from build123d import *

# Parameters (mm, degrees)
F1_DEPTH = 25
F8_DEPTH = 4
F9_R     = 2


with BuildPart() as f1:
    # F0 (on Top) → F1 (new body)
    with BuildSketch(Plane.XY):
        Polygon((0, -35), (30.3108891325, -17.5), (30.3108891325, 17.5), (0, 35), (-30.3108891325, 17.5), (-30.3108891325, -17.5), align=None)
    extrude(amount=F1_DEPTH)

    # F1_face (on face) → F3 section 0
    with BuildSketch(Plane.XY.offset(25)):
        Polygon((-30.3108891325, -17.5), (0, -35), (30.3108891325, -17.5), (30.3108891325, 17.5), (0, 35), (-30.3108891325, 17.5), align=None)
    # F2 (on Top) → F3 section 1
    with BuildSketch(Plane.XY):
        Polygon((43.3012701892, 25), (0, 50), (-43.3012701892, 25), (-43.3012701892, -25), (0, -50), (43.3012701892, -25), align=None)
    loft()

    # F4 (on Top) → F6 section 0
    with BuildSketch(Plane.XY):
        Polygon((-40.7031939779, -23.5), (0, -47), (40.7031939779, -23.5), (40.7031939779, 23.5), (0, 47), (-40.7031939779, 23.5), align=None)
    # F5 (on face) → F6 section 1
    with BuildSketch(Plane.XY.offset(25)):
        Polygon((27.7128129211, 16), (0, 32), (-27.7128129211, 16), (-27.7128129211, -16), (0, -32), (27.7128129211, -16), align=None)
    loft(mode=Mode.SUBTRACT)

    # F7 (on face) → F8 (join)
    with BuildSketch(Plane.XY.offset(25)):
        Polygon((-30.3108891325, -17.5), (0, -35), (30.3108891325, -17.5), (30.3108891325, 17.5), (0, 35), (-30.3108891325, 17.5), align=None)
    extrude(amount=-F8_DEPTH)

    # F9
    f9_edges = [f1.edges().sort_by_distance(p)[0] for p in [
        (-14.895637, -25.8, 21),
        (-29.791274, 0, 21),
        (14.895637, -25.8, 21),
        (29.791274, 0, 21),
        (14.895637, 25.8, 21),
        (-14.895637, 25.8, 21),
    ]]
    fillet(f9_edges, radius=F9_R)


solid = f1.part
The listing builds one solid part. Answer for the finished solid, in the listing's coordinates (mm). Give positions to 0.01 mm unless a question says otherwise; leave off trailing zeros.
1) For a pull along X with two mould halves and no side action, classify faces 1 (the face through (0, 0, 21)), 2 (the face through (22, 35, 0)) as pulls with the +X half, pulls with the -X half, needs draft (parallel to the pull), parting line crosses it, or undercut.
2) Given P1, Ø17, axis at x = -9.5, y = 2.5, coming from the -Z side; P2, Ø1.5, axis at x = 27.5, y = -36.5, coming from the -Z side; P3, Ø3, axis at x = 34, z = 7, coming from the -Y side; P4, Ø12, axis at x = -5.5, z = 22, coming from the -Y side, each flat-ended and moving along its own axis, determine where each tip first touches the part or whether it passes through.
3) Find the intervals of material crossed by L1, parallel to X at y = 7, z = 9.5; L2, parallel to X at y = 12, z = 20; L3, parallel to Y at x = 12, z = 5, in increasing order.
Response:
1. face 1: undercut
1. face 2: needs draft
2. P1: stops at z = 21
2. P2: passes through
2. P3: stops at y = -27.42
2. P4: stops at y = -38.62
3. L1: x = -38.36 to -35.77, 35.77 to 38.36
3. L2: x = -32.91 to -30.31, 30.31 to 32.91
3. L3: y = -40.07 to -37.07, 37.07 to 40.07
